```python
from build123d import *

# Parameters (mm, degrees)
F0_W     = 1.5
F0_H     = 5
F1_DEPTH = 25
F2_R     = 1.5
F3_DEPTH = 25
F4_W     = 4
F4_H     = 10
F5_DEPTH = 25
F6_R     = 0.25


with BuildPart() as f1:
    # F0 (on Top) → F1 (new body)
    with BuildSketch(Plane.XY):
        with BuildLine():
            ThreePointArc((3.570714, 1.5), (1.936492, 0.390228), (0, 0))
            Line((0, 0), (11.5, 0))
            ThreePointArc((11.5, 0), (15.035534, 1.464466), (16.5, 5))
            Line((16.5, 5), (15, 5))
            Line((15, 5), (13.5, 5))
            Line((13.5, 5), (13.5, 3.5))
            ThreePointArc((13.5, 3.5), (12.914214, 2.085786), (11.5, 1.5))
            Line((11.5, 1.5), (10, 1.5))
            Line((10, 1.5), (3.570714, 1.5))
        make_face()
        with Locations((14.25, 7.5)):
            Rectangle(F0_W, F0_H)
    extrude(amount=F1_DEPTH)

    # F2 (on face) → F3 (cut)
    with BuildSketch(Plane.YZ.offset(15)):
        with Locations((7.5, 12.5)):
            Circle(F2_R)
    extrude(amount=-F3_DEPTH, mode=Mode.SUBTRACT)

    # F4 (on face) → F5 (cut)
    with BuildSketch(Plane.XZ):
        with Locations((5, 13)):
            Rectangle(F4_W, F4_H)
    extrude(amount=-F5_DEPTH, mode=Mode.SUBTRACT)

    # F6
    f6_edges = [f1.edges().sort_by_distance(p)[0] for p in [
        (0, 0, 12.5),
    ]]
    fillet(f6_edges, radius=F6_R)


solid = f1.part
```
Work out the finished part from the listing and answer in its coordinate system (mm). A direction names the side the tool comes from. Round coordinates to 2 decimals unless told otherwise and drop trailing zeros. Write each loop counter-clockwise with the first axis right and the second up, starting at its lowest first coordinate (ties: lowest second). Pieces come first, ordered by that corner, then holes. Notation, with made-up numbers: (5.25, -22) -> (17.25, -22) arc R23 ccw to (17.25, 7) -> close; hole circle Ø6 at (-0.75, 38). An arc over 180 degrees is marked (long way). Write each question's results on one line, items separated by ' | '.
1) The part is cut by section B-B (z = 12.5). Write down the section's boundary in (x, y), and give its area (3 significant figures).
Findings:
outline: (2.13, 0.48) arc R0.25 ccw to (2.24, 0) -> (3, 0) -> (3, 1) arc R5 cw to start; (7, 0) -> (11.5, 0) arc R5 ccw to (16.5, 5) -> (15, 5) -> (15, 6) -> (13.5, 6) -> (13.5, 3.5) arc R2 cw to (11.5, 1.5) -> (7, 1.5) -> close; (13.5, 9) -> (15, 9) -> (15, 10) -> (13.5, 10) -> close | area: 23.9 mm²
2) Consider line 1 along Z through (x, y) = (14.05, 7.5); line 2 along Y through (x, z) = (5.25, 1); line 3 along X through (y, z) = (8.75, 6.75). Determine where each line is inside the solid, lowest interval first. Write a range as [from, to].
Findings:
line 1: z = [0, 11], [14, 25] | line 2: y = [0, 1.5] | line 3: x = [13.5, 15]
3) The part is cut by section A-A (z = 17.75). Write down the section's boundary in (x, y), and give its area (3 significant figures).
Findings:
outline: (2.13, 0.48) arc R0.25 ccw to (2.24, 0) -> (3, 0) -> (3, 1) arc R5 cw to start; (7, 0) -> (11.5, 0) arc R5 ccw to (16.5, 5) -> (15, 5) -> (15, 10) -> (13.5, 10) -> (13.5, 3.5) arc R2 cw to (11.5, 1.5) -> (7, 1.5) -> close | area: 28.4 mm²
4) The part is cut by section C-C (y = 7.5). Write down the section's boundary in (x, z).
Findings:
outline: (13.5, 0) -> (15, 0) -> (15, 11) -> (13.5, 11) -> close; (13.5, 14) -> (15, 14) -> (15, 25) -> (13.5, 25) -> close
5) The part is cut by section D-D (x = 6.75). Write down the section's boundary in (y, z), and give its area (3 significant figures).
Findings:
outline: (0, 0) -> (1.5, 0) -> (1.5, 8) -> (0, 8) -> close; (0, 18) -> (1.5, 18) -> (1.5, 25) -> (0, 25) -> close | area: 22.5 mm²
6) Flat-ended cylindrical pins translate along their axes: pin 1 (5 mm diameter, centred on y = 8, z = 9, fed in from -X); pin 2 (0.8 mm diameter, centred on y = 0.5, z = 12, fed in from -X); pin 3 (1 mm diameter, centred on x = 7, z = 5, fed in from +Y); pin 4 (0.8 mm diameter, centred on y = 0.5, z = 15, fed in from +X). Find the tip coordinate at first contact, or state that the pin passes through.
Findings:
pin 1: stops at x = 13.5 | pin 2: stops at x = 1.99 | pin 3: stops at y = 1.5 | pin 4: stops at x = 14.36
7) For a pull along Y with two mould halves and no side action, classify faces 1 (the flat face through (14, 3, 25)), 2 (the flat face through (8, 0, 12)), 3 (the flat face through (14, 10, 12)), 4 (the cylindrical face through (14.3, 6.3, 11.6)) as +Y half, -Y half, draft (parallel to the pull), parting line (faces both ways), or undercut.
Findings:
face 1: draft | face 2: -Y half | face 3: +Y half | face 4: undercut
8) Which of the six approach directions +Z, -Z, +X, -X, +Y, -Y give full straight-line access (tool end or side, diameter ignored) to faces 5 (the flat face through (7, 1, 13)), 6 (the cylindrical face through (15, 1.43, 12.32)), 7 (the flat face through (8, 1.5, 12)), 8 (the flat face through (14, 3, 0)), 9 (the flat face through (15, 5.8, 12.3))?
Findings:
face 5: +Y, -Y | face 6: +Z, -Z, +X, -Y | face 7: +Z, -Z, -X, +Y | face 8: -Z, +X, -X, +Y, -Y | face 9: +Z, -Z, +X, +Y
